The listing builds one solid part. Answer for the finished solid, in the listing's coordinates (mm). A direction names the side the tool comes from. Coordinates: 2 decimals unless noted, no trailing zeros. Loops run counter-clockwise (first coordinate to the right, second up) from the corner with the lowest first, then second, coordinate; pieces in that order, holes last. Notation, with made-up numbers: M -13.5,73 L 37.5,73 A8 ccw 37.5,86 Z; hole C 42,27 d6. An arc over 180 degrees is marked long. Return JSON: item names as keys, results as strings. Group by question number.
1. The mould has two halves that part along Z. Classify faces 4 (the face through (-56.144, -1.521, 35.019)), 5 (the face through (-42.061, -10, -32)), 6 (the face through (-44, -10, -68)): pulls with the +Z half, pulls with the -Z half, needs draft (parallel to the pull), parting line crosses it, or undercut.
2. Section C-C (x = -33) is taken. Write down the section's boundary in (y, z).
3. Given P1, Ø2, axis at x = -68, z = 50.5, coming from the -Y side; P2, Ø5, axis at y = -15.5, z = -8, coming from the -X side; P3, Ø2, axis at x = -78.5, z = 10.5, coming from the -Y side; P4, Ø12, axis at y = -17.5, z = 24.5, coming from the -X side, each flat-ended and moving along its own axis, determine where each tip first touches the part or whether it passes through.
4. Which of the six approach directions +Z, -Z, +X, -X, +Y, -Y give full straight-line access (tool end or side, diameter ignored) to faces 1 (the face through (-52, -3, 28)), 2 (the face through (-51, -20, -25)), 3 (the face through (-60.061, -10, -31))?
5. Section A-A (y = -1.5) is taken. Write down the section's boundary in (x, z), then the cut area to 3 significant figures.
6. Section B-B (y = -8.5) is taken. Write down the section's boundary in (x, z).
7. Straight lines are drawn through the part: L1, parallel to Y at x = -58, z = 37.5; L2, parallel to X at y = -10, z = -14; L3, parallel to Z at x = -44.5, y = -11.75. For each, find the intervals that lie inside material, in ascending order. Write a range as from..to.
8. Section D-D (z = 11) is taken. Write down the section's boundary in (x, y).
```python
from build123d import *

# Parameters (mm, degrees)
F1_DEPTH = 20
F2_DEPTH = 20
F3_DEPTH = 3
F4_R     = 5
F5_DEPTH = 100


with BuildPart() as f1:
    # F0 (on Front) → F1 (new body)
    with BuildSketch(Plane.XZ):
        with BuildLine():
            ThreePointArc((-42.2376775657, 0.9527799487), (-23.4282681394, 13.4322820603), (-16.1492416263, 34.7992572542))
            ThreePointArc((-16.1492416263, 34.7992572542), (-72.5162168202, 62.5202307411), (-60.0608056868, 0.9527799487))
            Line((-60.0608056868, 0.9527799487), (-54.3766204398, 0.9527799487))
            ThreePointArc((-54.3766204398, 0.9527799487), (-74.0213766418, 59.9560742196), (-17.1492416263, 34.7992572542))
            ThreePointArc((-17.1492416263, 34.7992572542), (-25.9924246609, 11.9271222387), (-47.9218628128, 0.9527799487))
            Line((-47.9218628128, 0.9527799487), (-42.2376775657, 0.9527799487))
        make_face()
    extrude(amount=F1_DEPTH)

    # F0 (on Front) → F2 (join)
    with BuildSketch(Plane.XZ):
        with BuildLine():
            ThreePointArc((-42.2376775657, 0.9527799487), (-51.1492416263, -0.2007427458), (-60.0608056868, 0.9527799487))
            Line((-60.0608056868, 0.9527799487), (-60.0608056868, -64.0472200513))
            ThreePointArc((-60.0608056868, -64.0472200513), (-58.5963395928, -67.5827539572), (-55.0608056868, -69.0472200513))
            Line((-55.0608056868, -69.0472200513), (-47.0608056868, -69.0472200513))
            ThreePointArc((-47.0608056868, -69.0472200513), (-43.5252717809, -67.5827539572), (-42.0608056868, -64.0472200513))
            Line((-42.0608056868, -64.0472200513), (-42.0608056868, 0.9527799487))
            Line((-42.0608056868, 0.9527799487), (-42.2376775657, 0.9527799487))
        make_face()
        with BuildLine():
            Line((-54.3766204398, 0.9527799487), (-60.0608056868, 0.9527799487))
            ThreePointArc((-60.0608056868, 0.9527799487), (-51.1492416263, -0.2007427458), (-42.2376775657, 0.9527799487))
            Line((-42.2376775657, 0.9527799487), (-47.9218628128, 0.9527799487))
            ThreePointArc((-47.9218628128, 0.9527799487), (-51.1492416263, 0.7992572542), (-54.3766204398, 0.9527799487))
        make_face()
    extrude(amount=F2_DEPTH)

    # F0 (on Front) → F3 (join)
    with BuildSketch(Plane.XZ):
        with BuildLine():
            ThreePointArc((-17.1492416263, 34.7992572542), (-74.0213766418, 59.9560742196), (-54.3766204398, 0.9527799487))
            Line((-54.3766204398, 0.9527799487), (-47.9218628128, 0.9527799487))
            ThreePointArc((-47.9218628128, 0.9527799487), (-25.9924246609, 11.9271222387), (-17.1492416263, 34.7992572542))
        make_face()
    extrude(amount=F3_DEPTH)

    # F4 (on face) → F5 (cut)
    with BuildSketch(Plane.XZ.offset(3)):
        with Locations((-51.1492416263, 34.7992572542)):
            Circle(F4_R)
    extrude(amount=-F5_DEPTH, mode=Mode.SUBTRACT)


solid = f1.part
```
Worked out:
{
 "1": {"face 4": "undercut", "face 5": "needs draft", "face 6": "pulls with the -Z half"},
 "2": {"outline": "M -20,4.87 L 0,4.87 L 0,64.73 L -20,64.73 L -20,63.55 L -3,63.55 L -3,6.05 L -20,6.05 Z"},
 "3": {"P1": "y = -3", "P2": "x = -60.06", "P3": "through", "P4": "x = -85.88"},
 "4": {"face 1": "-Y", "face 2": "+Z, -Z, +X, -X, -Y", "face 3": "-Z, -X, +Y, -Y"},
 "5": {"outline": "M -60.06,-64.05 A5 ccw -55.06,-69.05 L -47.06,-69.05 A5 ccw -42.06,-64.05 L -42.06,0.95 L -42.24,0.95 A35 ccw long -60.06,0.95 Z; hole C -51.15,34.8 d10; hole M -54.38,0.95 A34 ccw -47.92,0.95 Z", "area": "5,000 mm^2"},
 "6": {"outline": "M -60.06,-64.05 A5 ccw -55.06,-69.05 L -47.06,-69.05 A5 ccw -42.06,-64.05 L -42.06,0.95 L -42.24,0.95 A35 ccw long -60.06,0.95 Z; hole C -51.15,34.8 d68"},
 "7": {"L1": "-3..0", "L2": "-60.06..-42.06", "L3": "-68.34..1.46, 68.14..69.16"},
 "8": {"outline": "M -76.81,-20 L -75.43,-20 L -75.43,-3 L -26.87,-3 L -26.87,-20 L -25.49,-20 L -25.49,0 L -76.81,0 Z"}
}
